CAD build for the part. Positions are in the model's coordinates, mm. Coordinates: 2 decimals unless noted, no trailing zeros. Order: outer loops, then holes, each group sorted by start corner. A loop starts at its lowest first (then second) coordinate and runs counter-clockwise, first axis right, second up. Notation, with made-up numbers: (75.25, 10) - (89.25, 10) arc R30 ccw to (89.25, 42) - close; hole circle Ø8 at (0, 68.25). An arc over 180 degrees is marked (long way). Return JSON: item names as keys, results as strings.
from build123d import *

# Parameters (mm, degrees)
SKETCH1_R           = 2
BOSS_EXTRUDE1_DEPTH = 4


with BuildPart() as part:
    # Sketch1 → Boss-Extrude1 (new body)
    with BuildSketch(Plane(origin=(0, 0, 0), x_dir=(1, 0, 0), z_dir=(0, 1, 0))):
        with BuildLine():
            Line((9, -5), (9, 5))
            ThreePointArc((9, 5), (0, 8.61916848), (-9, 5))
            Line((-9, 5), (-9, -5))
            ThreePointArc((-9, -5), (0, -8.61916848), (9, -5))
        make_face()
        with Locations((-5, 0)):
            Circle(SKETCH1_R, mode=Mode.SUBTRACT)
    extrude(amount=BOSS_EXTRUDE1_DEPTH)


solid = part.part
Item 1: Band-saw the part on B-B, the plane x = -5. List the corners of the cut face in (y, z).
Findings below:
{"outline": "(0, -7.62) - (4, -7.62) - (4, -2) - (0, -2) - close; (0, 2) - (4, 2) - (4, 7.62) - (0, 7.62) - close"}
Item 2: Band-saw the part on D-D, the plane z = -5.5. List the corners of the cut face in (x, y).
Findings below:
{"outline": "(-8.45, 0) - (8.45, 0) - (8.45, 4) - (-8.45, 4) - close"}
Item 3: Band-saw the part on A-A, the plane z = 0. List the corners of the cut face in (x, y).
Findings below:
{"outline": "(-9, 0) - (-7, 0) - (-7, 4) - (-9, 4) - close; (-3, 0) - (9, 0) - (9, 4) - (-3, 4) - close"}
Item 4: Wall check: L1, parallel to X at y = 1.6, z = 0; L2, parallel to Z at x = -5, y = 2.6; L3, parallel to Z at x = 3.25, y = 1.4. Give the ranges that are in metal, low to high. Write a range as [from, to].
Findings below:
{"L1": "x = [-9, -7], [-3, 9]", "L2": "z = [-7.62, -2], [2, 7.62]", "L3": "z = [-8.21, 8.21]"}
Item 5: Mould opens along Z. For faces 1 (the cylindrical face through (0.14, 1.97, -8.62)), 2 (the cylindrical face through (-6.6, 2, 1.2)), 3 (the flat face through (-9, 2, 0)) say: released by +Z, released by -Z, zero draft, split by the parting line, or undercut.
Findings below:
{"face 1": "released by -Z", "face 2": "undercut", "face 3": "zero draft"}
Item 6: Drop flat-ended pins along their axis: P1, Ø1, axis at x = 5, y = 1, coming from the +Z side; P2, Ø3, axis at x = -5, z = 0, coming from the -Y side. Give the stop position or say it passes through.
Findings below:
{"P1": "stops at z = 7.82", "P2": "passes through"}
Item 7: Band-saw the part on C-C, the plane y = 3.3. List the corners of the cut face in (x, z), then the cut area to 3 significant figures.
Findings below:
{"outline": "(-9, -5) arc R13 ccw to (9, -5) - (9, 5) arc R13 ccw to (-9, 5) - close; hole circle Ø4 at (-5, 0)", "area": "257 mm²"}
